Here's the drawing with two shaded views (mm, measured from the low corner). I have some questions. A direction names the side the tool comes from. Coordinates: 2 decimals unless noted, no trailing zeros. Write each loop counter-clockwise with the first axis right and the second up, starting at its lowest first coordinate (ties: lowest second). Pieces come first, ordered by that corner, then holes. Notation, with made-up numbers: (20, -4) -> (75, -4) arc R6 cw to (75, 5) -> close; hole circle Ø6 at (43, 4). An arc over 180 degrees is marked (long way). Put each result on its own line as item: value. Start each with the question number.
Item 1: I want a section at B-B, the plane z = 11. List the corners of the cut face in (x, y) for me (1 decimal), then the cut area to 3 significant figures.
Item 2: If we mould it in two halves opening along Z, with no side actions, what happens to the marked faces 1, 2 and 3? For each: released by +Z, released by -Z, zero draft, split by the parting line, or undercut.
Item 3: I need wall thicknesses on line 1 (Y direction, x = 10.5, z = 72); line 2 (Y direction, x = 34, z = 36); line 3 (X direction, y = 8.5, z = 75) (1 decimal). Which ranges of each line are inside material? Lowest first, please. Write a range as [from, to].
Item 4: I want a section at C-C, the plane y = 5.5. List the corners of the cut face in (x, z) for me (1 decimal).
Item 5: I want a section at A-A, the plane x = 10. List the corners of the cut face in (y, z) for me (1 decimal), then the cut area to 3 significant figures.
Item 6: For pin 1 (1.5 mm diameter, centred on x = 60, y = 10.5, fed in from +Z); pin 2 (6 mm diameter, centred on y = 7, z = 45.5, fed in from -X); pin 3 (6 mm diameter, centred on y = 20, z = 65.5, fed in from -X); pin 4 (10 mm diameter, centred on x = 76.5, z = 27, fed in from -Y), each with a flat end and sliding along its axis, tell me the tip position at first contact or that it passes through.
Item 7: On a 3-axis mill with a long thin cutter (end or side, diameter ignored), from which of +Z, -Z, +X, -X, +Y, -Y can I reach the whole of each face in a straight line? I mean the marked faces 4, 5, 6, 7 and 8. Say none if no direction works.
Item 8: I want a section at D-D, the plane z = 56. List the corners of the cut face in (x, y) for me.
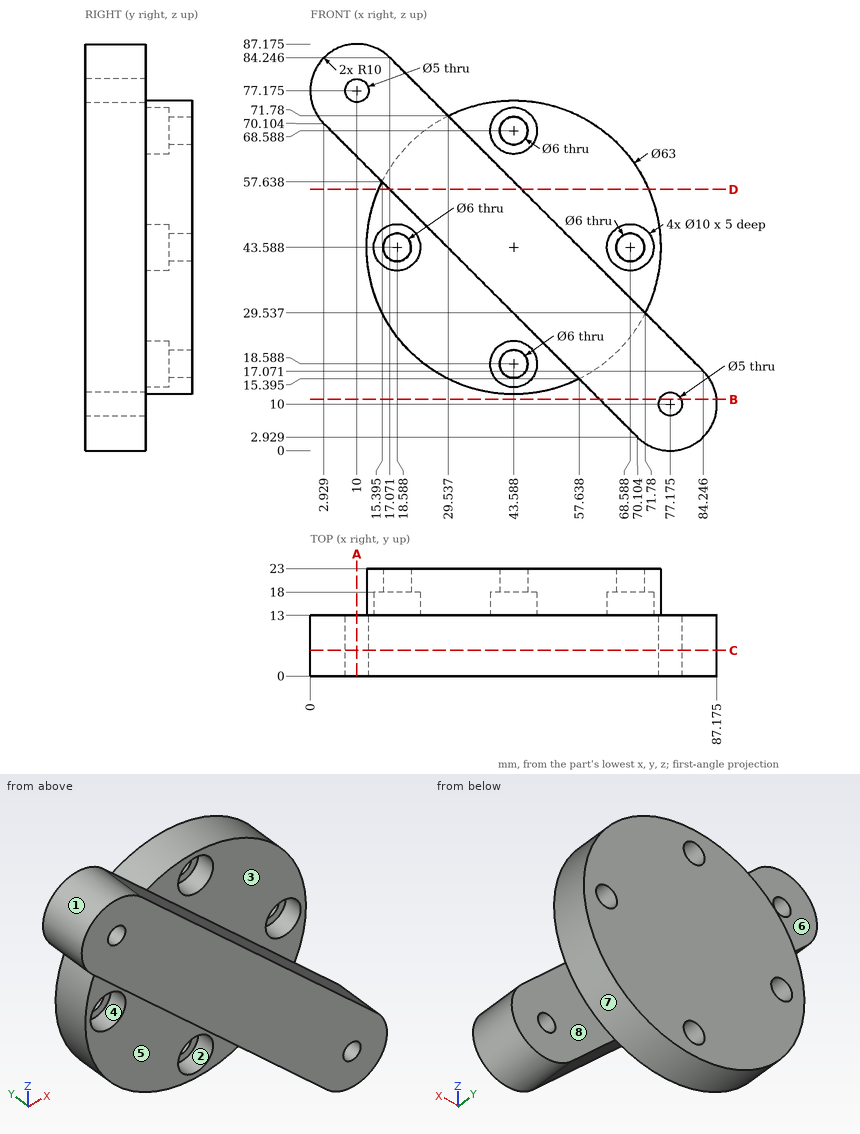
Calculated:
1. outline: (62, 0) -> (74.9, 0) -> (74.9, 13) -> (62, 13) -> close; (79.5, 0) -> (87.1, 0) -> (87.1, 13) -> (79.5, 13) -> close
1. area: 267 mm2
2. face 1: split by the parting line
2. face 2: undercut
2. face 3: zero draft
3. line 1: y = [0, 13]
3. line 2: y = [13, 23]
3. line 3: x = [0.2, 8.8], [11.2, 26.3]
4. outline: (2.9, 70.1) -> (70.1, 2.9) arc R10 ccw to (84.2, 17.1) -> (17.1, 84.2) arc R10 ccw to start; hole circle Ø5 at (10, 77.2); hole circle Ø5 at (77.2, 10)
5. outline: (0, 63) -> (13, 63) -> (13, 74.7) -> (0, 74.7) -> close; (0, 79.7) -> (13, 79.7) -> (13, 87.2) -> (0, 87.2) -> close
5. area: 249 mm2
6. pin 1: stops at z = 42.07
6. pin 2: stops at x = 24.53
6. pin 3: stops at x = 18.4
6. pin 4: stops at y = 0
7. face 4: -Y
7. face 5: -Z, -X, -Y
7. face 6: +Z, -X, +Y
7. face 7: +Y
7. face 8: -Z, +X, +Y
8. outline: (14.64, 13) -> (17.03, 13) -> (17.03, 0) -> (45.32, 0) -> (45.32, 13) -> (72.54, 13) -> (72.54, 23) -> (14.64, 23) -> close
